from build123d import *

# Parameters (mm, degrees)
SKETCH_R     = 3
PAD_DEPTH    = 54.5
SKETCH001_R  = 2
PAD001_DEPTH = 2
SKETCH002_R  = 3
PAD002_DEPTH = 1
SKETCH003_R  = 2
PAD003_DEPTH = 2
SKETCH004_R  = 3
PAD004_DEPTH = 1


with BuildPart() as part:
    # Sketch → Pad (new body)
    with BuildSketch(Plane.YZ):
        Circle(SKETCH_R)
    extrude(amount=PAD_DEPTH)

    # Sketch001 (on Face3 of Pad) → Pad001 (join)
    with BuildSketch(Plane.YZ.offset(54.5)):
        Circle(SKETCH001_R)
    extrude(amount=PAD001_DEPTH)

    # Sketch002 (on Face5 of Pad001) → Pad002 (join)
    with BuildSketch(Plane.YZ.offset(56.5)):
        Circle(SKETCH002_R)
    extrude(amount=PAD002_DEPTH)

    # Sketch003 (on Face7 of Pad002) → Pad003 (join)
    with BuildSketch(Plane(origin=(0, 0, 0), x_dir=(0, 1, 0), z_dir=(-1, 0, 0))):
        Circle(SKETCH003_R)
    extrude(amount=PAD003_DEPTH)

    # Sketch004 (on Face9 of Pad003) → Pad004 (join)
    with BuildSketch(Plane(origin=(-2, 0, 0), x_dir=(0, 1, 0), z_dir=(-1, 0, 0))):
        Circle(SKETCH004_R)
    extrude(amount=PAD004_DEPTH)


solid = part.part
Geometry check sheet. Reference: the model listing, model coordinates, mm. A direction names the side the tool comes from. Round coordinates to 2 decimals unless told otherwise and drop trailing zeros. Order: outer loops, then holes, each group sorted by start corner. A loop starts at its lowest first (then second) coordinate and runs counter-clockwise, first axis right, second up. Notation, with made-up numbers: M 36.5,-20 L 57.5,-20 A24 cw 57.5,16 Z; hole C 20.5,81 d2. An arc over 180 degrees is marked long. Answer in a Markdown table with one row per item.
(1) Sectioned sample at A-A, the plane y = 0. Record the cut outline in (x, z).
Responses:
| item | result |
|---|---|
| outline | M -3,-3 L -2,-3 L -2,-2 L 0,-2 L 0,-3 L 54.5,-3 L 54.5,-2 L 56.5,-2 L 56.5,-3 L 57.5,-3 L 57.5,3 L 56.5,3 L 56.5,2 L 54.5,2 L 54.5,3 L 0,3 L 0,2 L -2,2 L -2,3 L -3,3 Z |
(2) Tool access check on faces 1 (the face through (0, 1, -2)), 2 (the face through (57.5, 0, 0)). Record the directions out of +Z, -Z, +X, -X, +Y, -Y that give a thin tool (end or side, any length) a straight path to the whole face; none if there is none.
Responses:
| item | result |
|---|---|
| face 1 | none |
| face 2 | +Z, -Z, +X, +Y, -Y |
(3) Draft check along X on faces 3 (the face through (-2.5, -3, -0.1)), 4 (the face through (-3, 0, 0)), 5 (the face through (56.5, 1, -2)), 6 (the face through (-2, 1, 2)). Enter one of: released by +X, released by -X, zero draft, split by the parting line, or undercut.
Responses:
| item | result |
|---|---|
| face 3 | zero draft |
| face 4 | released by -X |
| face 5 | undercut |
| face 6 | undercut |
(4) Sectioned sample at C-C, the plane x = 47.5. Record the cut outline in (y, z).
Responses:
| item | result |
|---|---|
| outline | C 0,0 d6 |
(5) Scan lines: probe 1 along X at (y, z) = (2.4, 0.3); probe 2 along Y at (x, z) = (39.5, -1.65); probe 3 along Z at (x, y) = (37.5, -1.95). Record each from-to range of solid material in increasing order. Write a range as from..to.
Responses:
| item | result |
|---|---|
| probe 1 | x = -3..-2, 0..54.5, 56.5..57.5 |
| probe 2 | y = -2.51..2.51 |
| probe 3 | z = -2.28..2.28 |
(6) Go/stop test with a flat-tipped pin: P1, Ø1, axis at x = 19, z = 1.5, coming from the +Y side. Record where the tip stops, or that it passes through.
Responses:
| item | result |
|---|---|
| P1 | stops at y = 2.83 |
